from build123d import *

# Parameters (mm, degrees)
F0_W      = 127
F0_H      = 76.2
F1_DEPTH  = 50.8
F2_R      = 5.08
F3_W      = 7
F3_H      = 14.7
F4_DEPTH  = 16.4
F5_W      = 7
F5_H      = 14.3
F6_DEPTH  = 16.44
F7_W      = 7
F7_H      = 14.3
F8_DEPTH  = 25.4
F9_R      = 9.7907841867
F10_DEPTH = 1.27
F11_DEPTH = 22.352
F13_DEPTH = 25.4
F14_DEPTH = 25.4
F15_DEPTH = 25.4
F16_DEPTH = 10
F17_R     = 5.08


with BuildPart() as f1:
    # F0 (on Front) → F1 (new body)
    with BuildSketch(Plane.XZ):
        Rectangle(F0_W, F0_H)
    extrude(amount=F1_DEPTH)

    # F2
    f2_edges = [f1.edges().sort_by_distance(p)[0] for p in [
        (0, -50.8, 38.1),
        (0, 0, 38.1),
        (0, -50.8, -38.1),
        (0, 0, -38.1),
    ]]
    fillet(f2_edges, radius=F2_R)

    # F3 (on face) → F4 (join)
    with BuildSketch(Plane.YZ.offset(63.5)):
        with BuildLine():
            Line((-5.08, 38.1), (-45.72, 38.1))
            ThreePointArc((-45.72, 38.1), (-49.3121024484, 36.6121024484), (-50.8, 33.02))
            Line((-50.8, 33.02), (-50.8, -33.02))
            ThreePointArc((-50.8, -33.02), (-49.3121024484, -36.6121024484), (-45.72, -38.1))
            Line((-45.72, -38.1), (-5.08, -38.1))
            ThreePointArc((-5.08, -38.1), (-1.4878975516, -36.6121024484), (0, -33.02))
            Line((0, -33.02), (0, 33.02))
            ThreePointArc((0, 33.02), (-1.4878975516, 36.6121024484), (-5.08, 38.1))
        make_face()
        with Locations((-42.22, 25.675587382)):
            Rectangle(F3_W, F3_H, mode=Mode.SUBTRACT)
        with Locations((-42.22, 25.675587382)):
            Rectangle(F3_W, F3_H)
    extrude(amount=-F4_DEPTH)

    # F5 (on face) → F6 (join)
    with BuildSketch(Plane.YZ.offset(63.5)):
        with BuildLine():
            ThreePointArc((-50.8, -33.02), (-49.3121024484, -36.6121024484), (-45.72, -38.1))
            Line((-45.72, -38.1), (-5.08, -38.1))
            ThreePointArc((-5.08, -38.1), (-1.4878975516, -36.6121024484), (0, -33.02))
            Line((0, -33.02), (0, 33.02))
            ThreePointArc((0, 33.02), (-1.4878975516, 36.6121024484), (-5.08, 38.1))
            Line((-5.08, 38.1), (-45.72, 38.1))
            ThreePointArc((-45.72, 38.1), (-49.3121024484, 36.6121024484), (-50.8, 33.02))
            Line((-50.8, 33.02), (-50.8, -33.02))
        make_face()
        with Locations((-42.22, 25.4086919344)):
            Rectangle(F5_W, F5_H, mode=Mode.SUBTRACT)
    extrude(amount=F6_DEPTH)

    # F7 (on face) → F8 (join)
    with BuildSketch(Plane.YZ.offset(79.94)):
        with BuildLine():
            Line((-5.08, 38.1), (-45.72, 38.1))
            ThreePointArc((-45.72, 38.1), (-49.3121024484, 36.6121024484), (-50.8, 33.02))
            Line((-50.8, 33.02), (-50.8, -33.02))
            ThreePointArc((-50.8, -33.02), (-49.3121024484, -36.6121024484), (-45.72, -38.1))
            Line((-45.72, -38.1), (-5.08, -38.1))
            ThreePointArc((-5.08, -38.1), (-1.4878975516, -36.6121024484), (0, -33.02))
            Line((0, -33.02), (0, 33.02))
            ThreePointArc((0, 33.02), (-1.4878975516, 36.6121024484), (-5.08, 38.1))
        make_face()
        with Locations((-42.22, 25.4086919344)):
            Rectangle(F7_W, F7_H, mode=Mode.SUBTRACT)
        with BuildLine():
            Line((-35.5440098792, 20.9126272823), (-35.5440098792, 29.4131070442))
            ThreePointArc((-35.5440098792, 29.4131070442), (-34.6226893957, 31.6373714509), (-32.398424989, 32.5586919344))
            Line((-32.398424989, 32.5586919344), (-30.8212536197, 32.5586919344))
            ThreePointArc((-30.8212536197, 32.5586919344), (-28.6659921506, 31.6659534035), (-27.7732536197, 29.5106919344))
            Line((-27.7732536197, 29.5106919344), (-27.7732536197, 20.9126272823))
            ThreePointArc((-27.7732536197, 20.9126272823), (-28.6659921506, 18.7573658132), (-30.8212536197, 17.8646272823))
            Line((-30.8212536197, 17.8646272823), (-32.4960098792, 17.8646272823))
            ThreePointArc((-32.4960098792, 17.8646272823), (-34.6512713483, 18.7573658132), (-35.5440098792, 20.9126272823))
        make_face(mode=Mode.SUBTRACT)
    extrude(amount=F8_DEPTH)

    # F9 (on face) → F10 (join)
    with BuildSketch(Plane.XZ.offset(50.8)):
        with Locations((79.4515386224, 17.386501655)):
            Circle(F9_R)
    extrude(amount=F10_DEPTH)

    # F11 (add): a face of the model
    f11_faces = [f1.faces().sort_by_distance(p)[0] for p in [
        (79.4515386224, -52.07, 17.386501655),
    ]]
    extrude(f11_faces, amount=-F11_DEPTH)

    # F12 (on face) → F13 (join)
    with BuildSketch(Plane(origin=(-63.5, 0, 0), x_dir=(0, -1, 0), z_dir=(-1, 0, 0))):
        with BuildLine():
            Line((20.797392028, 16.5488310158), (19.2076092115, 16.5488310158))
            ThreePointArc((19.2076092115, 16.5488310158), (16.5135323752, 15.4329078521), (15.3976092115, 12.7388310158))
            Line((15.3976092115, 12.7388310158), (15.3976092115, 11.0805211589))
            Line((15.3976092115, 11.0805211589), (15.6854148954, 11.0805211589))
            Line((15.6854148954, 11.0805211589), (24.607392028, 11.0805211589))
            Line((24.607392028, 11.0805211589), (24.607392028, 12.7388310158))
            ThreePointArc((24.607392028, 12.7388310158), (23.4914688643, 15.4329078521), (20.797392028, 16.5488310158))
        make_face()
    extrude(amount=-F13_DEPTH)

    # F12 (on face) → F14 (join)
    with BuildSketch(Plane(origin=(-63.5, 0, 0), x_dir=(0, -1, 0), z_dir=(-1, 0, 0))):
        with BuildLine():
            Line((20.797392028, 16.5488310158), (19.2076092115, 16.5488310158))
            ThreePointArc((19.2076092115, 16.5488310158), (16.5135323752, 15.4329078521), (15.3976092115, 12.7388310158))
            Line((15.3976092115, 12.7388310158), (15.3976092115, 11.0805211589))
            Line((15.3976092115, 11.0805211589), (15.6854148954, 11.0805211589))
            Line((15.6854148954, 11.0805211589), (24.607392028, 11.0805211589))
            Line((24.607392028, 11.0805211589), (24.607392028, 12.7388310158))
            ThreePointArc((24.607392028, 12.7388310158), (23.4914688643, 15.4329078521), (20.797392028, 16.5488310158))
        make_face()
    extrude(amount=-F14_DEPTH)

    # F12 (on face) → F15 (join)
    with BuildSketch(Plane(origin=(-63.5, 0, 0), x_dir=(0, -1, 0), z_dir=(-1, 0, 0))):
        with BuildLine():
            Line((20.797392028, 16.5488310158), (19.2076092115, 16.5488310158))
            ThreePointArc((19.2076092115, 16.5488310158), (16.5135323752, 15.4329078521), (15.3976092115, 12.7388310158))
            Line((15.3976092115, 12.7388310158), (15.3976092115, 11.0805211589))
            Line((15.3976092115, 11.0805211589), (15.6854148954, 11.0805211589))
            Line((15.6854148954, 11.0805211589), (24.607392028, 11.0805211589))
            Line((24.607392028, 11.0805211589), (24.607392028, 12.7388310158))
            ThreePointArc((24.607392028, 12.7388310158), (23.4914688643, 15.4329078521), (20.797392028, 16.5488310158))
        make_face()
    extrude(amount=-F15_DEPTH)

    # F12 (on face) → F16 (join)
    with BuildSketch(Plane(origin=(-63.5, 0, 0), x_dir=(0, -1, 0), z_dir=(-1, 0, 0))):
        with BuildLine():
            ThreePointArc((50.8, 33.02), (49.3121024484, 36.6121024484), (45.72, 38.1))
            Line((45.72, 38.1), (5.08, 38.1))
            ThreePointArc((5.08, 38.1), (1.4878975516, 36.6121024484), (0, 33.02))
            Line((0, 33.02), (0, -33.02))
            ThreePointArc((0, -33.02), (1.4878975516, -36.6121024484), (5.08, -38.1))
            Line((5.08, -38.1), (45.72, -38.1))
            ThreePointArc((45.72, -38.1), (49.3121024484, -36.6121024484), (50.8, -33.02))
            Line((50.8, -33.02), (50.8, 33.02))
        make_face()
        with BuildLine():
            ThreePointArc((15.3976092115, 12.7388310158), (16.5135323752, 15.4329078521), (19.2076092115, 16.5488310158))
            Line((19.2076092115, 16.5488310158), (20.797392028, 16.5488310158))
            ThreePointArc((20.797392028, 16.5488310158), (23.4914688643, 15.4329078521), (24.607392028, 12.7388310158))
            Line((24.607392028, 12.7388310158), (24.607392028, 11.0805211589))
            Line((24.607392028, 11.0805211589), (15.6854148954, 11.0805211589))
            Line((15.6854148954, 11.0805211589), (15.3976092115, 11.0805211589))
            Line((15.3976092115, 11.0805211589), (15.3976092115, 12.7388310158))
        make_face(mode=Mode.SUBTRACT)
    extrude(amount=F16_DEPTH)

    # F17
    f17_edges = [f1.edges().sort_by_distance(p)[0] for p in [
        (-73.5, -25.4, 38.1),
        (-73.5, 0, 0),
        (-73.5, -25.4, -38.1),
        (-73.5, -50.8, 0),
        (-73.5, -49.312102, 36.612102),
        (-73.5, -1.487898, 36.612102),
        (-73.5, -49.312102, -36.612102),
        (-73.5, -1.487898, -36.612102),
    ]]
    fillet(f17_edges, radius=F17_R)


solid = f1.part
Work out the finished part from the listing and answer in its coordinate system (mm). A direction names the side the tool comes from. Round coordinates to 2 decimals unless told otherwise and drop trailing zeros. Loops run counter-clockwise (first coordinate to the right, second up) from the corner with the lowest first, then second, coordinate; pieces in that order, holes last. Notation, with made-up numbers: (31.5, -27.5) - (76.5, -27.5) arc R15 cw to (76.5, -23.5) - close; hole circle Ø6 at (4.25, -14.75). An arc over 180 degrees is marked (long way). Use one line per item in the form item = value. Start each with the question number.
(1) Find section D-D on z = -9. Determine the outline of the cut face in (x, y).
(2) Find section B-B on y = -42.5. Determine the outline of the cut face in (x, z).
(3) Consider line 1 (Y direction, x = 80, z = 28); line 2 (Y direction, x = -5, z = -17); line 3 (Z direction, x = 94, y = -4.5). Determine where each line is inside the solid, lowest interval first.
(4) Find section A-A on x = 93.5. Determine the outline of the cut face in (y, z), and give its area (3 significant figures).
(5) Which of the six approach directions +Z, -Z, +X, -X, +Y, -Y give full straight-line access (tool end or side, diameter ignored) to faces 1 (the face through (-68.43, -16.48, 15.4)), 2 (the face through (92, -27.773, 25)), 3 (the face through (84, -45.72, 27))?
(6) Determine the mould class of faces 4 (the face through (79.655, -42.269, 27.175)), 5 (the face through (86.449, -32.672, 24.234)), 6 (the face through (20, -50.8, 0)) for opening direction X: +X half, -X half, draft (parallel to the pull), parting line (faces both ways), or undercut.
(7) Find section C-C on x = 22. Determine the outline of the cut face in (y, z).
(8) Flat-ended cylindrical pins translate along their axes: P1, Ø8.5, axis at y = -32, z = 25.5, coming from the +X side; P2, Ø0.8, axis at x = -69, z = 12, coming from the -Y side; P3, Ø0.8, axis at x = -71, z = 12, coming from the +Y side. Find the tip coordinate at first contact, or state that the pin passes through.
Answer list:
q1.outline = (-73.5, -45.72) arc R5.08 ccw to (-68.42, -50.8) - (105.34, -50.8) - (105.34, 0) - (-68.42, 0) arc R5.08 ccw to (-73.5, -5.08) - close
q2.outline = (-73.5, -33.02) arc R5.08 ccw to (-68.42, -38.1) - (105.34, -38.1) - (105.34, 18.26) - (89.2, 18.26) arc R9.79 ccw to (69.7, 18.26) - (63.5, 18.26) - (63.5, 32.56) - (105.34, 32.56) - (105.34, 38.1) - (-68.42, 38.1) arc R5.08 ccw to (-73.5, 33.02) - close
q3.line_1 = -50.8 to -45.72, -38.72 to -35.54, -27.77 to 0
q3.line_2 = -50.8 to 0
q3.line_3 = -38.07 to 38.07
q4.outline = (-50.8, -33.02) arc R5.08 ccw to (-45.72, -38.1) - (-5.08, -38.1) arc R5.08 ccw to (0, -33.02) - (0, 33.02) arc R5.08 ccw to (-5.08, 38.1) - (-45.72, 38.1) arc R5.08 ccw to (-50.8, 33.02) - close; hole (-45.72, 18.26) - (-38.72, 18.26) - (-38.72, 32.56) - (-45.72, 32.56) - close; hole (-35.54, 20.91) arc R3.05 ccw to (-32.5, 17.86) - (-30.82, 17.86) arc R3.05 ccw to (-27.77, 20.91) - (-27.77, 29.51) arc R3.05 ccw to (-30.82, 32.56) - (-32.4, 32.56) arc R3.15 ccw to (-35.54, 29.41) - close
q4.area = 3,640 mm^2
q5.face_1 = -X
q5.face_2 = +X
q5.face_3 = none
q6.face_4 = undercut
q6.face_5 = +X half
q6.face_6 = draft
q7.outline = (-50.8, -33.02) arc R5.08 ccw to (-45.72, -38.1) - (-5.08, -38.1) arc R5.08 ccw to (0, -33.02) - (0, 33.02) arc R5.08 ccw to (-5.08, 38.1) - (-45.72, 38.1) arc R5.08 ccw to (-50.8, 33.02) - close
q8.P1 = 105.34
q8.P2 = -50.8
q8.P3 = -0.49
